Can you work these out from the model? Positions are in its coordinate system, mm. A direction names the side the tool comes from. Give positions to 0.01 mm unless a question says otherwise; leave off trailing zeros. Write each loop counter-clockwise with the first axis right and the second up, starting at its lowest first coordinate (ties: lowest second). Pieces come first, ordered by that corner, then holes.
1. Suppose I cut it at C-C (z = 64.5). Please give me the cut outline in (x, y).
2. Suppose I cut it at D-D (x = -7.75). Please give me the cut outline in (y, z), and give its area (3 significant figures).
3. Suppose I cut it at A-A (x = 0). Please give me the cut outline in (y, z), and give its area (3 significant figures).
4. If I drill on probe 1 along Z at (x, y) = (-6.25, 13.5); probe 2 along Z at (x, y) = (-2.75, 9); probe 3 along X at (y, z) = (-8.5, 46), over which ranges is the centre line in solid material (lowest first)?
5. On a 3-axis mill with a long thin cutter (end or side, diameter ignored), from which of +Z, -Z, +X, -X, +Y, -Y can I reach the whole of each face in a straight line? I mean faces 1 (the flat face through (0, 6, 86.5)), 2 (the flat face through (0, 14.5, 73)), 3 (the cylindrical face through (-0.54, 8.17, 81.43)). Say none if no direction works.
6. I'm going to push flat-ended pins straight in: pin 1 (1 mm diameter, centred on x = 7.5, y = -10, fed in from +Z); pin 2 (2 mm diameter, centred on y = 1, z = 56.5, fed in from -X); pin 3 (1.5 mm diameter, centred on y = 8.5, z = 20, fed in from +X); pin 4 (1.5 mm diameter, centred on x = 8, z = 22.5, fed in from +Y). Where does each tip first touch, or does it pass through?
7. Suppose I cut it at B-B (y = 5.73). Please give me the cut outline in (x, z), and give its area (3 significant figures).
Autodesk Inventor part; units mm, degrees
ref_plane "YZ Plane" through (0, 0, 0) normal (1, 0, 0) x (0, 1, 0)
ref_plane "XY Plane" through (0, 0, 0) normal (0, 0, 1) x (1, 0, 0)
sketch "Sketch1" plane through (0, 0, 0) normal (0, 0, 1) x (1, 0, 0)
  circle A0 centre (0, 0) radius 15
  dimension "d0" = 30
extrude "Extrusion1" add sketch "Sketch1" along normal blind 74
sketch "Sketch2" plane through (0, 0, 74) normal (0, 0, 1) x (1, 0, 0)
  circle A0 centre (0, 0) radius 15
  circle A1 centre (0, 5.73) radius 5
  dimension "d3" = 10
  dimension "d4" = 15.73
extrude "Extrusion2" add sketch "Sketch2" along normal blind 2.5 contours A1
sketch "Sketch3" plane through (0, 5.73, 76.5) normal (0, 0, 1) x (1, 0, 0)
  circle A0 centre (0, 0) radius 5
  circle A1 centre (0, 0) radius 2.5
  point P0 (0, -5.73)
  dimension "d7" = 5
extrude "Extrusion3" add sketch "Sketch3" along normal blind 10 contours A1
sketch "Sketch4" plane through (0, 0, 0) normal (0, 1, 0) x (-1, 0, 0)
  point P0 (0, 0)
ref_plane "Work Plane1" through (0, 15, 0) normal (0, 1, 0) x (-1, 0, 0)
sketch "Sketch5" plane through (0, 15, 0) normal (0, 1, 0) x (-1, 0, 0)
  line L0 (-5, 74) -> (5, 74)
  line L1 (5, 74) -> (5, 72)
  line L2 (5, 72) -> (-5, 72)
  line L3 (-5, 72) -> (-5, 74)
  line L4 (-15, 74) -> (15, 74)
  point P0 (0, 0)
  point P1 (0, 74)
  dimension "d11" = 10
  dimension "d12" = 2
extrude "Extrusion4" cut sketch "Sketch5" against normal blind 0.5
properties part number "Hjul Motor"
Checks:
1. outline: circle Ø30 at (0, 0)
2. outline: (-12.84, 0) - (12.84, 0) - (12.84, 74) - (-12.84, 74) - close
2. area: 1,900 mm2
3. outline: (-15, 0) - (15, 0) - (15, 72) - (14.5, 72) - (14.5, 74) - (10.73, 74) - (10.73, 76.5) - (8.23, 76.5) - (8.23, 86.5) - (3.23, 86.5) - (3.23, 76.5) - (0.73, 76.5) - (0.73, 74) - (-15, 74) - close
3. area: 2,290 mm2
4. probe 1: z = 0 to 74
4. probe 2: z = 0 to 76.5
4. probe 3: x = -12.36 to 12.36
5. face 1: +Z, +X, -X, +Y, -Y
5. face 2: +Z, +X, -X, +Y
5. face 3: +Z
6. pin 1: stops at z = 74
6. pin 2: stops at x = -15
6. pin 3: stops at x = 12.84
6. pin 4: stops at y = 13.13
7. outline: (-13.86, 0) - (13.86, 0) - (13.86, 74) - (5, 74) - (5, 76.5) - (2.5, 76.5) - (2.5, 86.5) - (-2.5, 86.5) - (-2.5, 76.5) - (-5, 76.5) - (-5, 74) - (-13.86, 74) - close
7. area: 2,130 mm2
